```python
from build123d import *

# Parameters (mm, degrees)
SKETCH_4_W          = 115
SKETCH_4_H          = 145
EXTRUDE_1_DEPTH     = 4
SKETCH_5_W          = 16
SKETCH_5_H          = 4
EXTRUDE_2_DEPTH     = 2
SKETCH_6_W          = 21
SKETCH_6_H          = 4
EXTRUDE_3_DEPTH     = 4.5
EXTRUDE_START       = -115
SKETCH_6_2_W        = 21
SKETCH_6_2_H        = 4
EXTRUDE_4_DEPTH     = 6.5
CUT_EXTRUDE_START   = -1.8
SKETCH_7_W          = 20.6
SKETCH_7_H          = 2.2
CUT_EXTRUDE_1_DEPTH = 159.577679245
CUT_EXTRUDE_2_DEPTH = 99.239961319


with BuildPart() as part:
    # 草图4 → 凸台-拉伸1 (new body)
    with BuildSketch(Plane(origin=(0, 0, 0), x_dir=(1, 0, 0), z_dir=(0, 1, 0))):
        Rectangle(SKETCH_4_W, SKETCH_4_H)
    extrude(amount=EXTRUDE_1_DEPTH)

    # 草图5 → 凸台-拉伸2 (add)
    with BuildSketch(Plane(origin=(0, 0, -72.5), x_dir=(-1, 0, 0), z_dir=(0, 0, -1))):
        with Locations((-49.5, 2)):
            Rectangle(SKETCH_5_W, SKETCH_5_H)
        with Locations((-16.5, 2)):
            Rectangle(SKETCH_5_W, SKETCH_5_H)
        with Locations((16.5, 2)):
            Rectangle(SKETCH_5_W, SKETCH_5_H)
        with Locations((49.5, 2)):
            Rectangle(SKETCH_5_W, SKETCH_5_H)
    extrude(amount=EXTRUDE_2_DEPTH)

    # 草图6 → 凸台-拉伸3 (add)
    with BuildSketch(Plane.ZY.offset(57.5)):
        with Locations((-43, 2)):
            Rectangle(SKETCH_6_W, SKETCH_6_H)
        with Locations((-1, 2)):
            Rectangle(SKETCH_6_W, SKETCH_6_H)
        with Locations((41, 2)):
            Rectangle(SKETCH_6_W, SKETCH_6_H)
    extrude(amount=EXTRUDE_3_DEPTH)

    # 草图6<2> → 凸台-拉伸4 (add)
    with BuildSketch(Plane.ZY.offset(57.5).offset(EXTRUDE_START)):
        with Locations((-43, 2)):
            Rectangle(SKETCH_6_2_W, SKETCH_6_2_H)
        with Locations((-1, 2)):
            Rectangle(SKETCH_6_2_W, SKETCH_6_2_H)
        with Locations((41, 2)):
            Rectangle(SKETCH_6_2_W, SKETCH_6_2_H)
    extrude(amount=-EXTRUDE_4_DEPTH)

    # 草图7 → 切除-拉伸1 (cut, through all)
    with BuildSketch(Plane.XY.offset(72.5).offset(CUT_EXTRUDE_START)):
        with Locations((31.5, 1.1)):
            Rectangle(SKETCH_7_W, SKETCH_7_H)
        with Locations((-31.5, 1.1)):
            Rectangle(SKETCH_7_W, SKETCH_7_H)
        Polygon((-21.2, 2.2), (-19, 2.2), (-21.2, 0), align=None)
        Polygon((-41.8, 2.2), (-41.8, 0), (-44, 2.2), align=None)
        Polygon((41.8, 2.2), (44, 2.2), (41.8, 0), align=None)
        Polygon((21.2, 2.2), (21.2, 0), (19, 2.2), align=None)
    extrude(amount=-CUT_EXTRUDE_1_DEPTH, mode=Mode.SUBTRACT)

    # 草图8 → 切除-拉伸2 (cut, through all)
    with BuildSketch(Plane.XZ.offset(-2.2)):
        Polygon((-49.65, -74.5), (-41.8, -54.5), (41.8, -54.5), (49.65, -74.5), align=None)
    extrude(amount=CUT_EXTRUDE_2_DEPTH, mode=Mode.SUBTRACT)


solid = part.part
```
Geometry: final body of the model. Coordinates: model frame, mm. A direction names the side the tool comes from. Round coordinates to 2 decimals unless told otherwise and drop trailing zeros. Order: outer loops, then holes, each group sorted by start corner. A loop starts at its lowest first (then second) coordinate and runs counter-clockwise, first axis right, second up. Notation, with made-up numbers: M -9,10 L 48,10 A5 ccw 48,18 Z; hole C 38,10.25 d5. An arc over 180 degrees is marked long. Use one line per item in the form item = value. Start each with the question number.
Q1. Cut plane B-B (x = -29). Return loops of the section in (y, z).
Q2. Cut plane A-A (z = -26.5). Return loops of the section in (x, y).
Q3. Mould query, pull axis Z, two halves, no side actions, for faces 6 (the face through (61, 2, 51.5)), 7 (the face through (-60, 2, -53.5)), 8 (the face through (57.5, 2, -22)). Classes: +Z half, -Z half, draft (parallel to the pull), parting line (faces both ways), or undercut.
Q4. Access query for faces 1 (the face through (46.54, 1.12, -66.58)), 2 (the face through (57.5, 2, 62)), 3 (the face through (-57.5, 2, 62)), 4 (the face through (-60, 2, 30.5)), 5 (the face through (57.5, 2, -64)). Directions: +Z, -Z, +X, -X, +Y, -Y. A direction counts if a zero-diameter tool reaches every point of the face in a straight line with its end or side. Return the directions, or none.
Q5. Pin query (flat end, axial travel): pin 1 Ø2 at (y, z) = (1.5, 21) entering from +X; pin 2 Ø1.2 at (y, z) = (3, 63) entering from -X; pin 3 Ø1.2 at (x, y) = (-60.5, 2.5) entering from +Z. Return the tip coordinate at first contact, or that it passes through.
Q6. Material intervals for line 1 (X direction, y = 0.75, z = 31); line 2 (X direction, y = 0.8, z = -31.5); line 3 (Y direction, x = 17, z = -65.5), sorted ascending. Write a range as [from, to].
Q7. Cut plane C-C (z = -2). Return loops of the section in (x, y), and give its area (3 significant figures).
Q8. Cut plane D-D (x = 15). Return loops of the section in (y, z), and give its area (3 significant figures).
Geometry results:
q1.outline = M 0,70.7 L 2.2,70.7 L 2.2,-72.5 L 4,-72.5 L 4,72.5 L 0,72.5 Z
q2.outline = M -57.5,0 L -41.8,0 L -44,2.2 L -19,2.2 L -21.2,0 L 21.2,0 L 19,2.2 L 44,2.2 L 41.8,0 L 57.5,0 L 57.5,4 L -57.5,4 Z
q3.face_6 = +Z half
q3.face_7 = -Z half
q3.face_8 = undercut
q4.face_1 = -Z, -Y
q4.face_2 = +Z, +X, +Y, -Y
q4.face_3 = +Z, -X, +Y, -Y
q4.face_4 = -X, +Y, -Y
q4.face_5 = -Z, +X, +Y, -Y
q5.pin_1 = 57.5
q5.pin_2 = -57.5
q5.pin_3 = 51.5
q6.line_1 = [-62, -42.55], [-20.45, 20.45], [42.55, 64]
q6.line_2 = [-57.5, -42.6], [-20.4, 20.4], [42.6, 57.5]
q6.line_3 = [2.2, 4]
q7.outline = M -62,0 L -41.8,0 L -44,2.2 L -19,2.2 L -21.2,0 L 21.2,0 L 19,2.2 L 44,2.2 L 41.8,0 L 64,0 L 64,4 L -62,4 Z
q7.area = 404 mm^2
q8.outline = M 0,-54.5 L 2.2,-54.5 L 2.2,-74.5 L 4,-74.5 L 4,72.5 L 0,72.5 Z
q8.area = 544 mm^2
